Verification items for this drawing (mm, ordinates from the low corner). Round coordinates to 2 decimals unless told otherwise and drop trailing zeros. Loops run counter-clockwise (first coordinate to the right, second up) from the corner with the lowest first, then second, coordinate; pieces in that order, holes last. Notation, with made-up numbers: M -1,-31 L 26,-31 A28 ccw 26,-5 Z; hole C -22.5,-31.75 d8. An arc over 180 degrees is marked long. One line per item, written item: value.
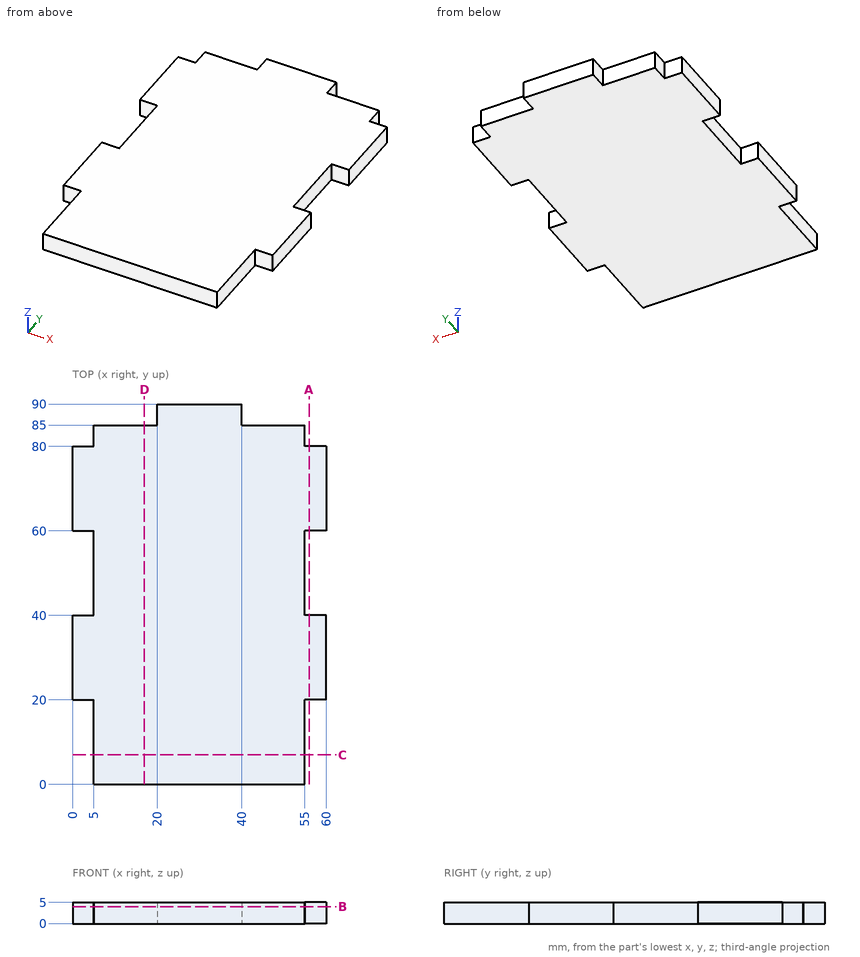
(1) Thickness scan on L1, parallel to X at y = 5, z = 1.25; L2, parallel to Y at x = 40.5, z = 1.45. Record the ranges inside material, lowest first. Write a range as from..to.
Completed:
L1: x = 5..55
L2: y = 0..85
(2) Sectioned sample at D-D on x = 17. Enter the section's corners in (y, z), and give its area (3 significant figures).
Completed:
outline: M 0,0 L 85,0 L 85,5 L 0,5 Z
area: 425 mm^2
(3) Sectioned sample at C-C on y = 7. Enter the section's corners in (x, z), and give its area (3 significant figures).
Completed:
outline: M 5,0 L 55,0 L 55,5 L 5,5 Z
area: 250 mm^2
(4) Depth check by flat-ended pin: pin 1 Ø1.5 at (y, z) = (57, 2.5) entering from +X; pin 2 Ø1.5 at (x, z) = (56.5, 3) entering from +Y; pin 3 Ø2 at (y, z) = (15.5, 1) entering from -X. Enter the tip coordinate at first touch or a pass-through.
Completed:
pin 1: stops at x = 55
pin 2: stops at y = 80
pin 3: stops at x = 5
(5) Sectioned sample at A-A on x = 56. Enter the section's corners in (y, z), and give its area (3 significant figures).
Completed:
outline: M 20,0 L 40,0 L 40,5 L 20,5 Z; M 60,0 L 80,0 L 80,5 L 60,5 Z
area: 200 mm^2
(6) Sectioned sample at B-B on z = 4. Enter the section's corners in (x, y).
Completed:
outline: M 0,20 L 5,20 L 5,0 L 55,0 L 55,20 L 60,20 L 60,40 L 55,40 L 55,60 L 60,60 L 60,80 L 55,80 L 55,85 L 40,85 L 40,90 L 20,90 L 20,85 L 5,85 L 5,80 L 0,80 L 0,60 L 5,60 L 5,40 L 0,40 Z
